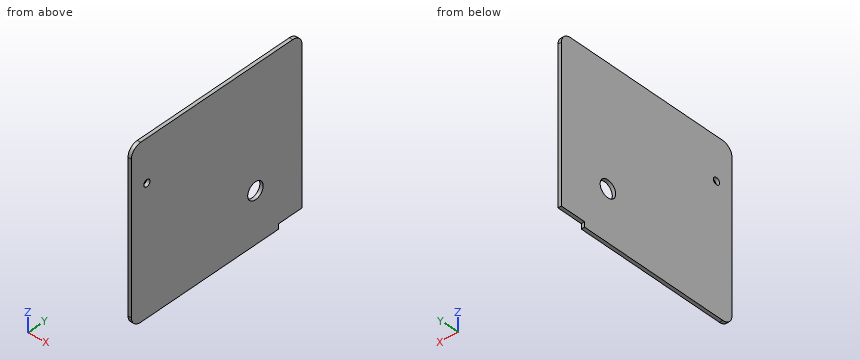
Autodesk Inventor part; units mm, degrees
ref_plane "YZ Plane" through (0, 0, 0) normal (1, 0, 0) x (0, 1, 0)
ref_plane "XZ Plane" through (0, 0, 0) normal (0, 1, 0) x (-1, 0, 0)
ref_plane "XY Plane" through (0, 0, 0) normal (0, 0, 1) x (1, 0, 0)
sketch "Sketch1" plane through (0, 0, 0) normal (1, 0, 0) x (0, 1, 0)
  line L0 (0, 0) -> (110, 0)
  line L1 (110, 0) -> (110, -100)
  line L2 (110, -100) -> (0, -100)
  line L3 (0, -100) -> (0, 0)
  line L4 (110, -97) -> (95, -97)
  line L5 (95, -97) -> (95, -100)
  line L6 (95, -100) -> (110, -100)
  line L7 (110, -100) -> (110, -97)
  circle A0 centre (10, -25) radius 2
  circle A1 centre (80, -70) radius 5
  point P0 (102.5, -100)
  point P1 (102.5, -97)
  point P2 (110, -98.5)
  point P3 (95, -98.5)
  dimension "d0" = 110
  dimension "d1" = 100
  dimension "d2" = 3
  dimension "d3" = 15
  dimension "d4" = 4
  dimension "d5" = 10
  dimension "d6" = 25
  dimension "d9" = 10
  dimension "d10" = 30
  dimension "d11" = 30
extrude "Plate2" add sketch "Sketch1" along normal blind 2 contours L0 L1 L4 L5 L2 L3
fillet "Corner Round2" radius 6 3 edges at (1, 110, 0) (1, 0, 0) (1, 0, -100)
equation "\"d12\" = Thickness"
equation "\"BendRadius\" = Thickness"
equation "\"BendReliefWidth\" = Thickness"
equation "\"BendReliefDepth\" = 0.5 * Thickness"
equation "\"CornerReliefSize\" = 4 * Thickness"
equation "\"MinimumRemnant\" = 2 * Thickness"
equation "\"TransitionRadius\" = BendRadius"
equation "\"JacobiRadiusSize\" = BendRadius"
equation "\"GapSize\" = Thickness"
properties part number "WI-Cover" material "Steel"
Here's how the part is built. I have some questions about the finished solid (model axes, mm). Round coordinates to 2 decimals unless told otherwise and drop trailing zeros. Loops run counter-clockwise (first coordinate to the right, second up) from the corner with the lowest first, then second, coordinate; pieces in that order, holes last. Notation, with made-up numbers: (23, -22) -> (80, -22) arc R5 ccw to (80, -15) -> close; hole circle Ø1 at (-10.5, -2). An arc over 180 degrees is marked (long way). Write each question's results on one line, items separated by ' | '.
(1) If we section it at A-A, the plane y = 10: List the corners of the cut face in (x, z) for me, then the cut area to 3 significant figures.
Worked answers:
outline: (0, -100) -> (2, -100) -> (2, -27) -> (0, -27) -> close; (0, -23) -> (2, -23) -> (2, 0) -> (0, 0) -> close | area: 192 mm2
(2) For P1, Ø3, axis at y = 18, z = -60.5, coming from the -X side; P2, Ø8, axis at y = 80, z = -70, coming from the -X side; P3, Ø1, axis at x = 1, z = -99, coming from the +Y side, each with a flat end and sliding along its axis, tell me the tip position at first contact or that it passes through.
Worked answers:
P1: x = 0 | P2: through | P3: y = 95
(3) If I drill on L1, parallel to Z at x = 1.55, y = 10; L2, parallel to Z at x = 0.7, y = 80; L3, parallel to Y at x = 1.75, z = -96, over which ranges is the centre line in solid material (lowest first)?
Worked answers:
L1: -100 to -27, -23 to 0 | L2: -100 to -75, -65 to 0 | L3: 0.34 to 110
(4) If we section it at B-B, the plane z = -25: List the corners of the cut face in (x, y) for me.
Worked answers:
outline: (0, 0) -> (2, 0) -> (2, 8) -> (0, 8) -> close; (0, 12) -> (2, 12) -> (2, 110) -> (0, 110) -> close
